Geometry check sheet. Reference: the model listing, model coordinates, mm. Face numbers are marked on the shaded views. A direction names the side the tool comes from. Round coordinates to 2 decimals unless told otherwise and drop trailing zeros. Order: outer loops, then holes, each group sorted by start corner. A loop starts at its lowest first (then second) coordinate and runs counter-clockwise, first axis right, second up. Notation, with made-up numbers: (84, 28.25) -> (122, 28.25) arc R19 ccw to (122, 32.25) -> close; hole circle Ø10 at (85, -11.5). An arc over 180 degrees is marked (long way). Use a Markdown table: item, result. Add a question column.
Item 1: Sectioned sample at A-A, the plane y = -31. Record the cut outline in (x, z), and give its area (3 significant figures).
Item 2: Set-up check for the marked faces 5, 6 and 7: record each of +Z, -Z, +X, -X, +Y, -Y from which the full face is reachable in a straight line by a thin tool's end or side.
Item 3: Gauge pin test, flat ends, axial feed: pin 1 Ø10 at (x, y) = (30, 15) entering from -Z; pin 2 Ø12.5 at (x, y) = (-12, -13.5) entering from +Z; pin 3 Ø6 at (x, z) = (-19.5, 108) entering from -Y. Record the tip position at first contact, or that the pin passes through.
Item 4: Mould release check, pull along Z, two halves, no side actions. Record for the marked faces 1, 2, 3 and 4: pulls with the +Z half, pulls with the -Z half, needs draft (parallel to the pull), parting line crosses it, or undercut.
Item 5: Material ranges on probe 1 along Z at (x, y) = (4, -27.5); probe 2 along Y at (x, z) = (33.5, 25); probe 3 along Y at (x, z) = (15.5, 16.5), recorded low to high. Write a range as [from, to].
from build123d import *

# Parameters (mm, degrees)
F0_W      = 76.2
F0_H      = 88.9
F1_DEPTH  = 127
F4_R      = 10.16
F5_DEPTH  = 76.201
F7_DEPTH  = 93.98
F10_DEPTH = 239.014
F11_R     = 10.16


with BuildPart() as f1:
    # F0 (on Top) → F1 (new body)
    with BuildSketch(Plane.XY):
        Rectangle(F0_W, F0_H)
    extrude(amount=F1_DEPTH)

    # F4
    f4_edges = [f1.edges().sort_by_distance(p)[0] for p in [
        (-38.1, -44.45, 63.5),
        (38.1, -44.45, 63.5),
    ]]
    fillet(f4_edges, radius=F4_R)

    # F3 (on face) → F5 (cut, through all)
    with BuildSketch(Plane.YZ.offset(38.1)):
        Polygon((-45.809648931, 49.2461211979), (7.4780625291, 49.2461211979), (22.2772937268, 93.8081741333), (16.8910045177, 99.4559377432), (22.2772937268, 129.883646965), (-45.809648931, 129.883646965), align=None)
    extrude(amount=-F5_DEPTH, mode=Mode.SUBTRACT)

    # F6 (on face) → F7 (cut)
    with BuildSketch(Plane(origin=(-38.1, 0, 0), x_dir=(0, -1, 0), z_dir=(-1, 0, 0))):
        with BuildLine():
            add(Edge.make_bspline(
                [(-48.9771775901, 121.8602433801), (-46.9556517053, 122.0553146871), (-45.5208898805, 120.6970387614), (-44.45, 118.2441702513)],
                knots=[0, 0, 0, 0, 0.0422373961, 0.0422373961, 0.0422373961, 0.0422373961], degree=3))
            add(Edge.make_bspline(
                [(-41.446827352, 0), (-59.6918978557, -6.5861209891), (-127.8152635251, 4.6198323194), (-62.2027540723, 120.584014117), (-48.9771775901, 121.8602433801)],
                knots=[0.5271103159, 0.5271103159, 0.5271103159, 0.5271103159, 0.7236671981, 1, 1, 1, 1], degree=3))
            Line((-41.446827352, 0), (-44.45, 0))
            Line((-44.45, 0), (-44.45, 118.2441702513))
        make_face()
    extrude(amount=-F7_DEPTH, mode=Mode.SUBTRACT)

    # F9 (on offset) → F10 (cut)
    with BuildSketch(Plane.YZ.offset(-192.024)):
        with BuildLine():
            add(Edge.make_bspline(
                [(58.8335432112, 110.7725277543), (50.7674633443, 117.1402640213), (25.8725163169, 57.9043750617), (12.2630217786, 9.8618308242), (73.8166292381, -18.5103461722), (69.968843038, 101.9818073895), (58.8335432112, 110.7725277543)],
                knots=[0, 0, 0, 0, 0.243523168, 0.4811201123, 0.6638139549, 1, 1, 1, 1], degree=3))
        make_face()
    extrude(amount=F10_DEPTH, mode=Mode.SUBTRACT)

    # F11
    f11_edges = [f1.edges().sort_by_distance(p)[0] for p in [
        (0, 16.891005, 99.455938),
        (-38.1, 14.877678, 71.527148),
        (38.1, 14.877678, 71.527148),
        (-38.1, -13.405969, 49.246121),
        (-38.1, 19.328919, 113.227969),
        (-38.1, 19.584149, 96.632056),
        (38.1, 19.584149, 96.632056),
        (38.1, 19.328919, 113.227969),
        (0, 21.766833, 127),
    ]]
    fillet(f11_edges, radius=F11_R)


solid = f1.part
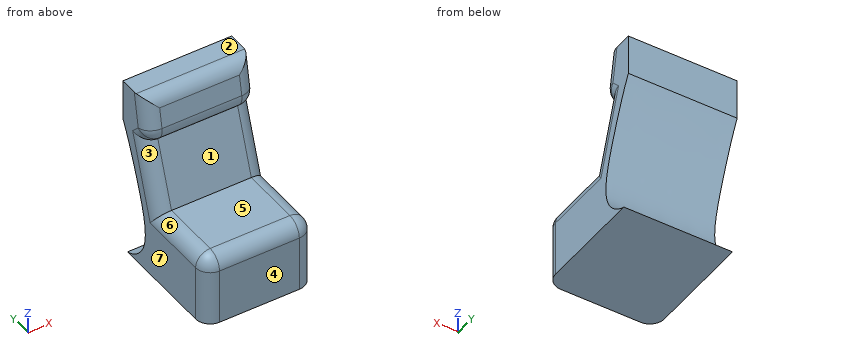
Found:
| question | item | result |
|---|---|---|
| 1 | outline | (-38.1, 0) -> (38.1, 0) -> (38.1, 39.09) arc R10.16 ccw to (27.94, 49.25) -> (-27.94, 49.25) arc R10.16 ccw to (-38.1, 39.09) -> close |
| 1 | area | 3,710 mm2 |
| 2 | face 5 | +Z, +X, -X, -Y |
| 2 | face 6 | +Z, -X, -Y |
| 2 | face 7 | +Z, -Z, -X, +Y, -Y |
| 3 | pin 1 | stops at z = 0 |
| 3 | pin 2 | stops at z = 49.25 |
| 3 | pin 3 | stops at y = 17.87 |
| 4 | face 1 | undercut |
| 4 | face 2 | pulls with the +Z half |
| 4 | face 3 | undercut |
| 4 | face 4 | needs draft |
| 5 | probe 1 | z = [0, 49.25] |
| 5 | probe 2 | y = [-42.79, 20.18] |
| 5 | probe 3 | y = [-44.45, 21.75] |
